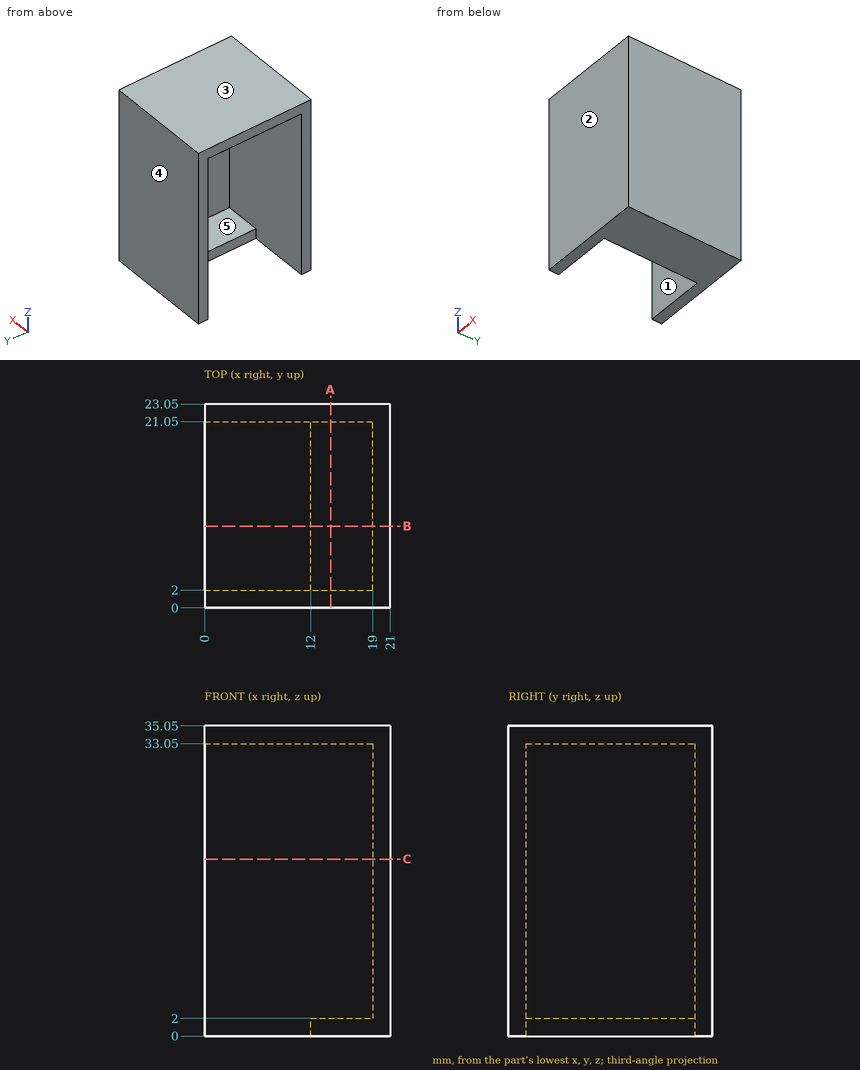
Geometry: see drawing. Coordinates: mm, zero at the bounding-box minimum. A direction names the side the tool comes from. Give positions to 0.01 mm unless a question says otherwise; leave off trailing zeros. Loops run counter-clockwise (first coordinate to the right, second up) from the corner with the lowest first, then second, coordinate; pieces in that order, holes last. Notation, with made-up numbers: (-35, 53.25) - (-22, 53.25) arc R19 ccw to (-22, 85.25) - close; hole circle Ø7 at (52, 33.25). An arc over 180 degrees is marked (long way). Use CSV: the item, a comma, the result in double quotes. Start each with the question number.
Item 1: Mould query, pull axis Y, two halves, no side actions, for the marked faces 3, 4 and 5. Classes: pulls with the +Y half, pulls with the -Y half, needs draft (parallel to the pull), parting line crosses it, or undercut.
Item 2: Section A-A on x = 14.25. Return loops of the section in (y, z), then the cut area to 3 significant figures.
Item 3: Section C-C on z = 20. Return loops of the section in (x, y), then the cut area to 3 significant figures.
Item 4: Section B-B on y = 9.25. Return loops of the section in (x, z), then the cut area to 3 significant figures.
Item 5: Line query: line 1 (Y direction, x = 13, z = 31); line 2 (Z direction, x = 17, y = 12); line 3 (Z direction, x = 2.25, y = 13.75). Output: solid intervals per line, ascending.
Item 6: Reachability of the marked faces 1 and 2 from +Z, -Z, +X, -X, +Y, -Y: full face, straight path, thin tool, end or side. Return the list, or none.
Item 7: Contact query for flat-ended pins moving along their axis: P1, Ø5.5, axis at y = 7.5, z = 23, coming from the -X side; P2, Ø9.5, axis at x = 13, y = 7, coming from the -Z side; P3, Ø1.6, axis at y = 7, z = 1.5, coming from the -X side. Output: stop coordinate, or through.
Ans:
1,face 3,"needs draft"
1,face 4,"pulls with the +Y half"
1,face 5,"undercut"
2,outline,"(0, 0) - (23.05, 0) - (23.05, 35.05) - (0, 35.05) - close; hole (2, 2) - (21.05, 2) - (21.05, 33.05) - (2, 33.05) - close"
2,area,"216 mm2"
3,outline,"(0, 0) - (21, 0) - (21, 23.05) - (0, 23.05) - (0, 21.05) - (19, 21.05) - (19, 2) - (0, 2) - close"
3,area,"122 mm2"
4,outline,"(0, 33.05) - (19, 33.05) - (19, 2) - (12, 2) - (12, 0) - (21, 0) - (21, 35.05) - (0, 35.05) - close"
4,area,"122 mm2"
5,line 1,"y = 0 to 2, 21.05 to 23.05"
5,line 2,"z = 0 to 2, 33.05 to 35.05"
5,line 3,"z = 33.05 to 35.05"
6,face 1,"-X"
6,face 2,"+Z, -Z, +X, -X, -Y"
7,P1,"stops at x = 19"
7,P2,"stops at z = 0"
7,P3,"stops at x = 12"
